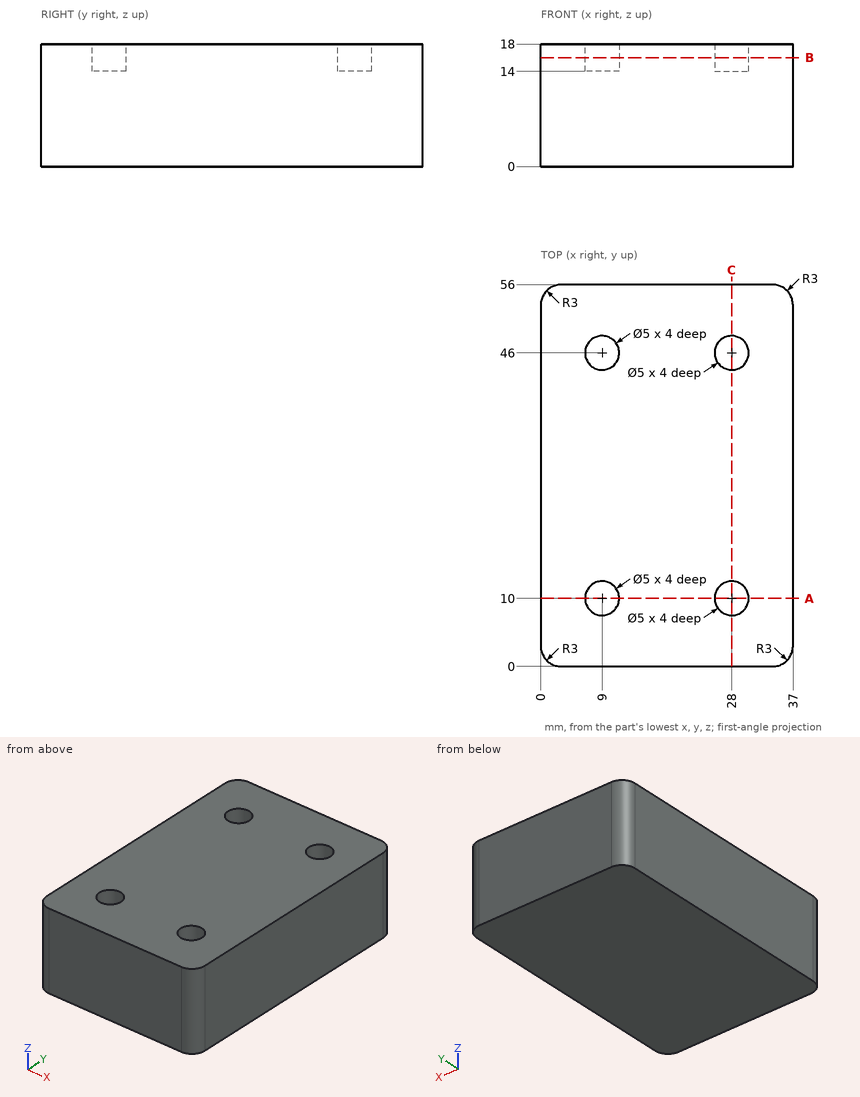
Study the drawing (mm; zero at the part's minimum x, y, z) and answer. Round coordinates to 2 decimals unless told otherwise and drop trailing zeros. Loops run counter-clockwise (first coordinate to the right, second up) from the corner with the lowest first, then second, coordinate; pieces in that order, holes last. Notation, with made-up numbers: (8, 35) - (30, 35) arc R29 ccw to (30, 63) - close; hole circle Ø1 at (7, -10). An arc over 180 degrees is marked (long way). Use one line per item in the form item = value. Start each with the question number.
1. The part is cut by section A-A on y = 10. Determine the outline of the cut face in (x, z), then the cut area to 3 significant figures.
2. Consider line 1 (Y direction, x = 9, z = 16.45); line 2 (Z direction, x = 26, y = 46); line 3 (Y direction, x = 2.5, z = 7.5). Determine where each line is inside the solid, lowest interval first. Write a range as [from, to].
3. The part is cut by section B-B on z = 16. Determine the outline of the cut face in (x, y), then the cut area to 3 significant figures.
4. The part is cut by section C-C on x = 28. Determine the outline of the cut face in (y, z), then the cut area to 3 significant figures.
5. Given pin 1 Ø4.5 at (x, y) = (28, 10) entering from +Z, flat-ended and moving along its own axis, determine where the tip first touches the part or whether it passes through.
Geometry check:
q1.outline = (0, 0) - (37, 0) - (37, 18) - (30.5, 18) - (30.5, 14) - (25.5, 14) - (25.5, 18) - (11.5, 18) - (11.5, 14) - (6.5, 14) - (6.5, 18) - (0, 18) - close
q1.area = 626 mm^2
q2.line_1 = [0, 7.5], [12.5, 43.5], [48.5, 56]
q2.line_2 = [0, 14]
q2.line_3 = [0.04, 55.96]
q3.outline = (0, 3) arc R3 ccw to (3, 0) - (34, 0) arc R3 ccw to (37, 3) - (37, 53) arc R3 ccw to (34, 56) - (3, 56) arc R3 ccw to (0, 53) - close; hole circle Ø5 at (9, 10); hole circle Ø5 at (9, 46); hole circle Ø5 at (28, 10); hole circle Ø5 at (28, 46)
q3.area = 1,990 mm^2
q4.outline = (0, 0) - (56, 0) - (56, 18) - (48.5, 18) - (48.5, 14) - (43.5, 14) - (43.5, 18) - (12.5, 18) - (12.5, 14) - (7.5, 14) - (7.5, 18) - (0, 18) - close
q4.area = 968 mm^2
q5.pin_1 = 14
